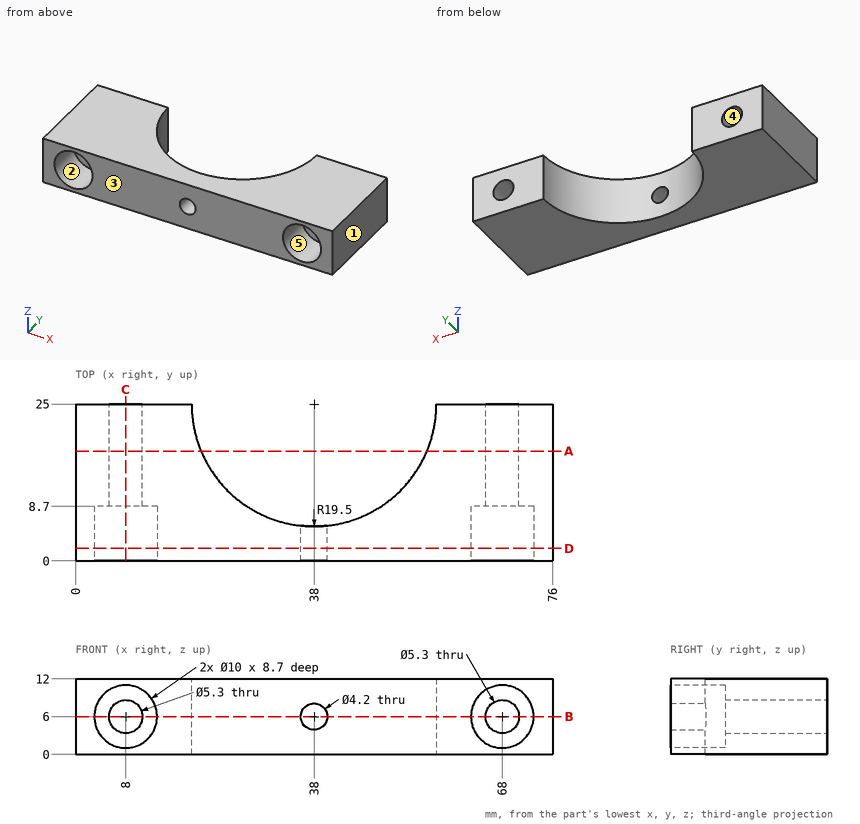
Geometry check sheet. Reference: drawing and pictorial views, mm from the part's lowest x, y, z. A direction names the side the tool comes from. Coordinates: 2 decimals unless noted, no trailing zeros. Order: outer loops, then holes, each group sorted by start corner. A loop starts at its lowest first (then second) coordinate and runs counter-clockwise, first axis right, second up. Notation, with made-up numbers: M -30,36.25 L 12,36.25 A33 ccw 12,68.25 Z; hole C 84,32.25 d10. An arc over 180 degrees is marked long. Write each question's results on one line, items separated by ' | '. Start each with the question number.
1. Cross-section at C-C on x = 8. Record the cut outline in (y, z).
2. Cross-section at B-B on z = 6. Record the cut outline in (x, y), and give its area (3 significant figures).
3. Cross-section at A-A on y = 17.5. Record the cut outline in (x, z).
4. Go/stop test with flat-tipped pins: P1, Ø6, axis at x = 68, z = 6, coming from the +Y side; P2, Ø5, axis at x = 8, z = 6.5, coming from the -Y side; P3, Ø5, axis at x = 53, z = 5, coming from the +Y side. Record where each tip stops, or that it passes through.
5. Material ranges on probe 1 along X at (y, z) = (20.5, 4); probe 2 along Z at (x, y) = (8, 17); probe 3 along X at (y, z) = (18.75, 4.5), recorded low to high.
6. Mould release check, pull along X, two halves, no side actions. Record for the marked faces 1, 2 and 3: +X half, -X half, draft (parallel to the pull), parting line (faces both ways), or undercut.
7. Access from +Z, -Z, +X, -X, +Y, -Y to the whole of each face (thin tool, end or side, straight path). Record for the marked faces 4 and 5.
8. Cross-section at D-D on y = 2. Record the cut outline in (x, z).
Checks:
1) outline: M 0,0 L 25,0 L 25,3.35 L 8.7,3.35 L 8.7,1 L 0,1 Z; M 0,11 L 8.7,11 L 8.7,8.65 L 25,8.65 L 25,12 L 0,12 Z
2) outline: M 0,0 L 3,0 L 3,8.7 L 5.35,8.7 L 5.35,25 L 0,25 Z; M 10.65,8.7 L 13,8.7 L 13,0 L 35.9,0 L 35.9,5.61 A19.5 cw 18.5,25 L 10.65,25 Z; M 40.1,0 L 63,0 L 63,8.7 L 65.35,8.7 L 65.35,25 L 57.5,25 A19.5 cw 40.1,5.61 Z; M 70.65,8.7 L 73,8.7 L 73,0 L 76,0 L 76,25 L 70.65,25 Z | area: 933 mm²
3) outline: M 0,0 L 20,0 L 20,12 L 0,12 Z; M 56,0 L 76,0 L 76,12 L 56,12 Z; hole C 8,6 d5.3; hole C 68,6 d5.3
4) P1: stops at y = 25 | P2: stops at y = 8.7 | P3: stops at y = 16.4
5) probe 1: x = 0 to 6.26, 9.74 to 19.03, 56.97 to 66.26, 69.74 to 76 | probe 2: z = 0 to 3.35, 8.65 to 12 | probe 3: x = 0 to 5.82, 10.18 to 19.53, 56.47 to 65.82, 70.18 to 76
6) face 1: +X half | face 2: undercut | face 3: draft
7) face 4: +Y, -Y | face 5: -Y
8) outline: M 0,0 L 76,0 L 76,12 L 0,12 Z; hole C 8,6 d10; hole C 38,6 d4.2; hole C 68,6 d10
